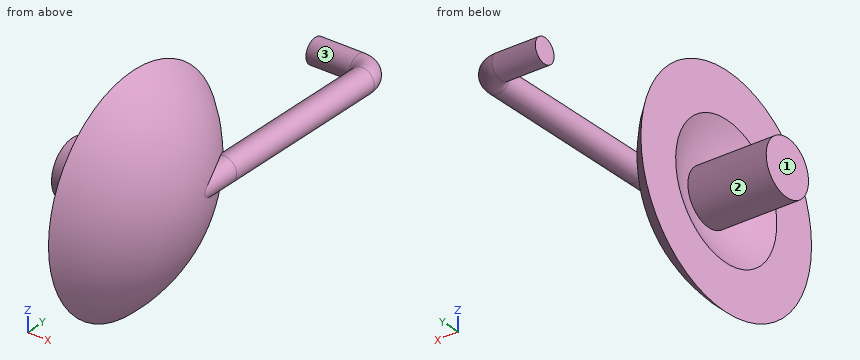
from build123d import *

# Parameters (mm, degrees)
SHELL3_T                        = -59.766763848
SKETCH6_R                       = 53.790087464
BOSS_EXTRUDE2_DEPTH             = 120
BOSS_EXTRUDE2_DIRECTION_2_REACH = 102
SKETCH5_R                       = 23.906705539
BOSS_EXTRUDE3_REACH             = 358.953


with BuildPart() as part:
    # Sketch2 → Revolve1 (revolve)
    with BuildSketch(Plane(origin=(0, 0, 0), x_dir=(1, 0, 0), z_dir=(0, 1, 0))):
        with BuildLine():
            Line((0, 0), (0, -216.95335277))
            ThreePointArc((0, -216.95335277), (73.796884119, -119.4453403), (100, 0))
            Line((100, 0), (0, 0))
        make_face()
    revolve(axis=Axis((100, 0, 0), (-1, 0, 0)))

    # Shell3
    shell3_openings = [part.faces().sort_by_distance(p)[0] for p in [
        (0, 0, -216.95335277),
    ]]
    offset(amount=SHELL3_T, openings=shell3_openings, kind=Kind.INTERSECTION)

    # Sketch6 → Boss-Extrude2 (add)
    with BuildSketch(Plane.ZY):
        Circle(SKETCH6_R)
    extrude(amount=BOSS_EXTRUDE2_DEPTH)

    # Sketch6 → Boss-Extrude2 direction 2 (add, up to next)
    with BuildSketch(Plane.ZY, mode=Mode.PRIVATE) as boss_extrude2_direction_2_sk1:
        Circle(SKETCH6_R)
    boss_extrude2_direction_2_tool1 = extrude(boss_extrude2_direction_2_sk1.sketch, amount=-BOSS_EXTRUDE2_DIRECTION_2_REACH, mode=Mode.PRIVATE) - part.part
    add(boss_extrude2_direction_2_tool1.solids().sort_by_distance((0, 0, 0))[0])

    # Sweep2: sweep along a path in Sketch4
    with BuildLine(Plane.XY) as sweep2_path:
        Line((75, 140), (75, 490))
        ThreePointArc((75, 490), (64.748737342, 514.748737342), (40, 525))
        Line((40, 525), (-45, 525))
    # Sketch5 → Sweep2 (sweep)
    with BuildSketch(Plane(origin=(0, 140, 0), x_dir=(1, 0, 0), z_dir=(0, 1, 0))):
        with Locations((70, 0)):
            Circle(SKETCH5_R)
    sweep(path=sweep2_path.line)

    # Sketch7 → Boss-Extrude3 (add, up to next)
    with BuildSketch(Plane.XZ.offset(-140), mode=Mode.PRIVATE) as boss_extrude3_sk1:
        with BuildLine():
            ThreePointArc((62.263560743, -22.620302327), (93.906705539, 0), (62.263560743, 22.620302327))
            ThreePointArc((62.263560743, 22.620302327), (63.29465881, 0), (62.263560743, -22.620302327))
        make_face()
    boss_extrude3_tool1 = extrude(boss_extrude3_sk1.sketch, amount=BOSS_EXTRUDE3_REACH, mode=Mode.PRIVATE) - part.part
    add(boss_extrude3_tool1.solids().sort_by_distance((76.458638, 140, 0))[0])


solid = part.part
The listing builds one solid part. Answer for the finished solid, in the listing's coordinates (mm). Face numbers are marked on the shaded views. Round coordinates to 2 decimals unless told otherwise and drop trailing zeros. Order: outer loops, then holes, each group sorted by start corner. A loop starts at its lowest first (then second) coordinate and runs counter-clockwise, first axis right, second up. Notation, with made-up numbers: (4, 52.5) -> (38, 52.5) arc R23 cw to (38, 60.5) -> close; hole circle Ø9 at (75.25, -32.5). An arc over 180 degrees is marked (long way). Put each result on its own line as item: value.
Q1. Determine the mould class of the marked faces 1, 2 and 3 for opening direction Y: pulls with the +Y half, pulls with the -Y half, needs draft (parallel to the pull), parting line crosses it, or undercut.
Results list:
face 1: needs draft
face 2: undercut
face 3: undercut
Q2. Each of these flat-tipped pins is pushed along its axis until it touches: P1, Ø5, axis at x = -76.5, z = 23, coming from the +Y side; P2, Ø4, axis at y = -50.5, z = -70.5, coming from the +X side; P3, Ø5, axis at y = -16, z = 62, coming from the +X side. Where does it stop, or does it pass through?
Results list:
P1: y = 49.73
P2: x = 87.13
P3: x = 93.29
Q3. Section C-C, the plane x = -99.5 is taken. Write down the section's boundary in (y, z).
Results list:
outline: circle Ø107.58 at (0, 0)
Q4. Section A-A, the plane z = -31.5 is taken. Write down the section's boundary in (x, y).
Results list:
outline: (-120, -43.6) -> (33.73, -43.6) arc R223.37 cw to (0, -124.66) -> (0, -214.65) arc R283.6 ccw to (0, 214.65) -> (0, 124.66) arc R223.37 cw to (33.73, 43.6) -> (-120, 43.6) -> close
Q5. Section B-B, the plane y = 0 is taken. Write down the section's boundary in (x, z), and give its area (3 significant figures).
Results list:
outline: (-120, -53.79) -> (33.73, -53.79) arc R225.58 cw to (0, -128.58) -> (0, -216.95) arc R285.34 ccw to (0, 216.95) -> (0, 128.58) arc R225.58 cw to (33.73, 53.79) -> (-120, 53.79) -> close
area: 40,100 mm^2
Q6. Section D-D, the plane y = 180.5 is taken. Write down the section's boundary in (x, z).
Results list:
outline: (0, -120.37) arc R221 ccw to (0, 120.37) -> close; circle Ø47.81 at (70, 0)
Q7. Consider line 1 along Z through (x, y) = (5.5, 11.5); line 2 along Z through (x, y) = (72.5, 152); line 3 along Z through (x, y) = (60, 347). Determine where each line is inside the solid, lowest interval first.
Results list:
line 1: -211.82 to -119.71, -52.55 to 52.55, 119.71 to 211.82
line 2: -23.78 to 23.78
line 3: -21.71 to 21.71
